Model file for the job. Use its own axes, mm. Face numbers are marked on the shaded views. A direction names the side the tool comes from. Round coordinates to 2 decimals unless told otherwise and drop trailing zeros. Order: outer loops, then holes, each group sorted by start corner. A loop starts at its lowest first (then second) coordinate and runs counter-clockwise, first axis right, second up. Notation, with made-up numbers: M 70.5,-29.5 L 115.5,-29.5 A10 ccw 115.5,-12.5 Z; hole C 71.25,39.5 d9. An arc over 180 degrees is marked long. Return JSON: item names as keys, results as strings. Group by question number.
Item 1: Slice it at C-C on y = 16.75. Write the cut outline in (x, z), then the cut area to 3 significant figures.
Item 2: Probe line 1 along Y through (x, z) = (-0.9, -1.35); line 2 along Y through (x, z) = (0.4, 0.2); line 3 along Z through (x, y) = (-0.2, 11.75). List the from-to ranges inside material, lowest first.
Item 3: Slice it at B-B on z = 0. Write the cut outline in (x, y).
Item 4: Slice it at A-A on x = 0. Write the cut outline in (y, z), then the cut area to 3 significant figures.
Item 5: Which spindle directions (+Z, -Z, +X, -X, +Y, -Y) get a long thin tool onto all of the face, cutting with end or side? Do the marked faces 1 and 2. Say none if no direction does.
Item 6: Slice it at D-D on y = 14. Write the cut outline in (x, z).
from build123d import *

# Parameters (mm, degrees)
CROQUIS1_R              = 2.05
SALIENTE_EXTRUIR1_DEPTH = 15.4
CROQUIS2_R              = 1.25
SALIENTE_EXTRUIR2_DEPTH = 2.8


with BuildPart() as part:
    # Croquis1 → Saliente-Extruir1 (new body)
    with BuildSketch(Plane(origin=(0, 0, 0), x_dir=(1, 0, 0), z_dir=(0, 1, 0))):
        Circle(CROQUIS1_R)
    extrude(amount=SALIENTE_EXTRUIR1_DEPTH)

    # Croquis2 → Saliente-Extruir2 (add)
    with BuildSketch(Plane(origin=(0, 15.4, 0), x_dir=(1, 0, 0), z_dir=(0, 1, 0))):
        Circle(CROQUIS2_R)
    extrude(amount=SALIENTE_EXTRUIR2_DEPTH)

    # Croquis4 → Revolución2 (revolve)
    with BuildSketch(Plane.XZ):
        with BuildLine():
            Line((0, -2.05), (0, 2.05))
            ThreePointArc((0, 2.05), (2.05, 0), (0, -2.05))
        make_face()
    revolve(axis=Axis((0, 0, -2.05), (0, 0, 1)))


solid = part.part
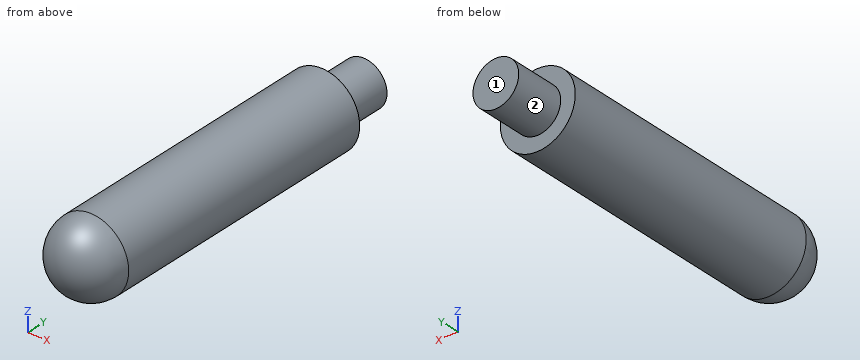
Output values:
{
 "1": {"outline": "C 0,0 d2.5", "area": "4.91 mm²"},
 "2": {"line 1": "-1.25 to 15.4", "line 2": "-2 to 18.2", "line 3": "-2.04 to 2.04"},
 "3": {"outline": "M -2.05,0 A2.05 ccw 2.05,0 L 2.05,15.4 L 1.25,15.4 L 1.25,18.2 L -1.25,18.2 L -1.25,15.4 L -2.05,15.4 Z"},
 "4": {"outline": "M 0,-2.05 L 15.4,-2.05 L 15.4,-1.25 L 18.2,-1.25 L 18.2,1.25 L 15.4,1.25 L 15.4,2.05 L 0,2.05 A2.05 ccw Z", "area": "76.7 mm²"},
 "5": {"face 1": "+Z, -Z, +X, -X, +Y", "face 2": "+Y"},
 "6": {"outline": "C 0,0 d4.1"}
}
